Can you work these out from the drawing? Everything is in mm from the part's minimum corner. A direction names the side the tool comes from. Give positions to 0.01 mm unless a question says otherwise; leave off trailing zeros. Order: outer loops, then holes, each group sorted by start corner. A loop starts at its lowest first (then second) coordinate and runs counter-clockwise, first axis right, second up. Notation, with made-up numbers: M -10,-7 L 43,-7 A19 ccw 43,-3 Z; hole C 14,-36.5 d5. An arc over 180 degrees is marked long. Use a Markdown table: item, result. Add a question column.
Item 1: Suppose I cut it at C-C on z = 17.5. Write out the boundary of the cut face in (x, y), plus the area to 3 significant figures.
Item 2: I'm going to push flat-ended pins straight in: pin 1 Ø3.5 at (x, y) = (2.05, 6.25) entering from +Z; pin 2 Ø2.5 at (x, y) = (2, 8.5) entering from -Z; pin 3 Ø7.5 at (y, z) = (9, 24.5) entering from -X. Where does each tip first touch, or does it pass through?
Item 3: Suppose I cut it at A-A on y = 6.25. Write out the boundary of the cut face in (x, z), plus the area to 3 significant figures.
Item 4: Suppose I cut it at B-B on x = 29.75. Write out the boundary of the cut face in (y, z).
Item 5: For the marked faces 1, 2 and 3, which set-ups out of +Z, -Z, +X, -X, +Y, -Y let a thin tool reach every point of the face, with its end or its side?
Item 6: Suppose I cut it at D-D on y = 10.25. Write out the boundary of the cut face in (x, z), plus the area to 3 significant figures.
Item 7: If I drill on L1, parallel to Y at x = 2.05, z = 17.75; L2, parallel to Z at x = 4.5, y = 10.5; L3, parallel to Z at x = 18, y = 2, over which ranges is the centre line in solid material (lowest first)? Write a range as from..to.
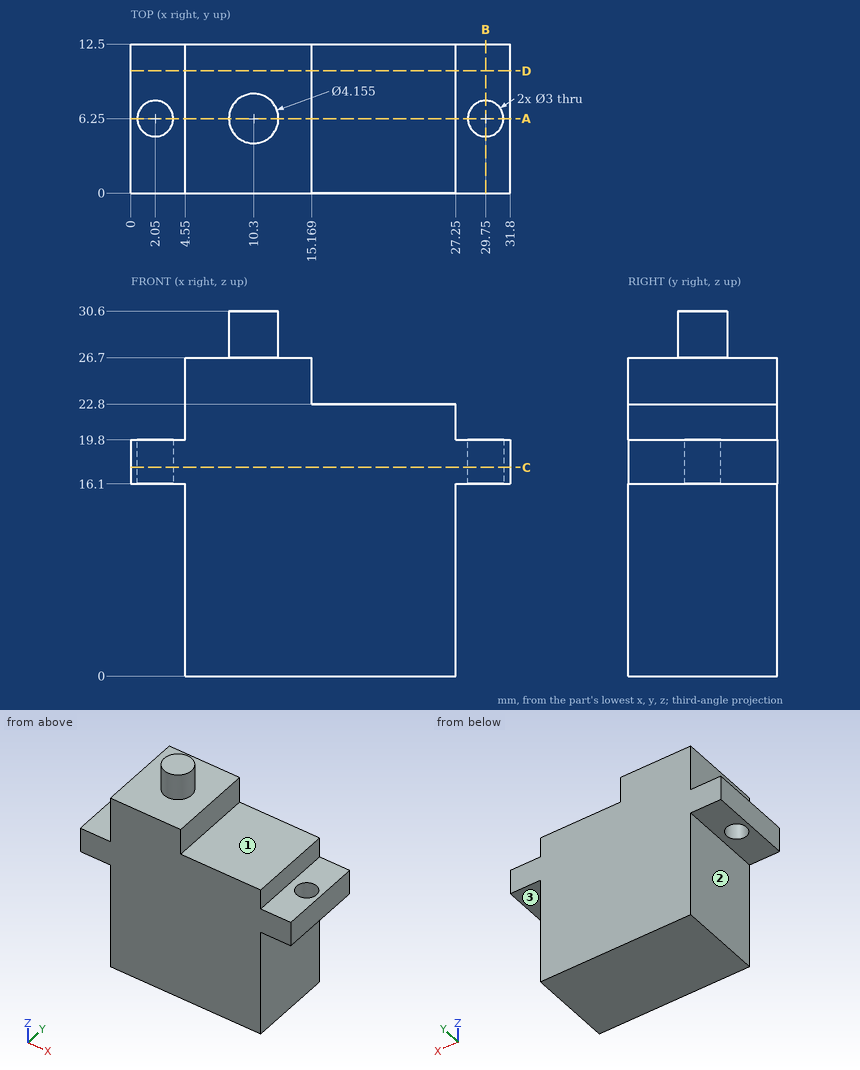
Findings below:
| question | item | result |
|---|---|---|
| 1 | outline | M 0,0 L 31.8,0 L 31.8,12.5 L 0,12.5 Z; hole C 2.05,6.25 d3; hole C 29.75,6.25 d3 |
| 1 | area | 383 mm^2 |
| 2 | pin 1 | stops at z = 19.8 |
| 2 | pin 2 | stops at z = 16.1 |
| 2 | pin 3 | stops at x = 4.55 |
| 3 | outline | M 0,16.1 L 0.55,16.1 L 0.55,19.8 L 0,19.8 Z; M 3.55,16.1 L 4.55,16.1 L 4.55,0 L 27.25,0 L 27.25,16.1 L 28.25,16.1 L 28.25,19.8 L 27.25,19.8 L 27.25,22.8 L 15.17,22.8 L 15.17,26.7 L 12.38,26.7 L 12.38,30.6 L 8.22,30.6 L 8.22,26.7 L 4.55,26.7 L 4.55,19.8 L 3.55,19.8 Z; M 31.25,16.1 L 31.8,16.1 L 31.8,19.8 L 31.25,19.8 Z |
| 3 | area | 587 mm^2 |
| 4 | outline | M 0,16.1 L 4.75,16.1 L 4.75,19.8 L 0,19.8 Z; M 7.75,16.1 L 12.5,16.1 L 12.5,19.8 L 7.75,19.8 Z |
| 5 | face 1 | +Z, +X, +Y, -Y |
| 5 | face 2 | -Z, -X, +Y, -Y |
| 5 | face 3 | -Z, +X, +Y, -Y |
| 6 | outline | M 0,16.1 L 4.55,16.1 L 4.55,0 L 27.25,0 L 27.25,16.1 L 31.8,16.1 L 31.8,19.8 L 27.25,19.8 L 27.25,22.8 L 15.17,22.8 L 15.17,26.7 L 4.55,26.7 L 4.55,19.8 L 0,19.8 Z |
| 6 | area | 593 mm^2 |
| 7 | L1 | y = 0..4.75, 7.75..12.5 |
| 7 | L2 | z = 16.1..19.8 |
| 7 | L3 | z = 0..22.8 |
